Geometry: final body of the model. Coordinates: model frame, mm. Give positions to 0.01 mm unless a question says otherwise; leave off trailing zeros. Loops run counter-clockwise (first coordinate to the right, second up) from the corner with the lowest first, then second, coordinate; pieces in that order, holes last.
from build123d import *

# Parameters (mm, degrees)
SKETCH1_W               = 544
SKETCH1_H               = 376
BOSS_EXTRUDE1_DEPTH     = 5
SKETCH2_R               = 6.5
SKETCH2_R_2             = 3
F_1_JOYYSTICK_DEPTH     = 6
SKETCH3_R               = 12.5
F_1_BUTTONS_DEPTH       = 6
SKETCH4_R               = 6.75
F_1_ROCKET_SWITCH_DEPTH = 6
SKETCH5_R               = 2.4
SKETCH5_W               = 2
SKETCH5_H               = 74
F_1_POTENTIOMETER_DEPTH = 6
FILLET1_R               = 35
SKETCH6_R               = 12.5
F_2_BUTTONS_DEPTH       = 6
SKETCH9_R               = 25
F_2_SPEAKER_DEPTH       = 6
SKETCH8_R               = 2.4
SKETCH8_W               = 2
SKETCH8_H               = 75
F_2_POTENTIOMETER_DEPTH = 6
SKETCH11_R              = 1.8
F_2_PCB1_DEPTH          = 6
SKETCH12_R              = 1.8
F_1_PCB2_DEPTH          = 6
SKETCH13_R              = 1.8
F_2_USB_CONNECTOR_DEPTH = 6
SKETCH14_R              = 1.8
F_1_USB_CONNECTOR_DEPTH = 6
SKETCH15_R              = 3
POWER_DEPTH             = 6
SKETCH16_R              = 1.8
LED_FIXINGS_DEPTH       = 6
SKETCH10_R              = 6.75
CUT_EXTRUDE1_DEPTH      = 6


with BuildPart() as part:
    # Sketch1 → Boss-Extrude1 (new body)
    with BuildSketch(Plane(origin=(0, 0, 0), x_dir=(1, 0, 0), z_dir=(0, 1, 0))):
        with Locations((272, 188)):
            Rectangle(SKETCH1_W, SKETCH1_H)
    extrude(amount=BOSS_EXTRUDE1_DEPTH)

    # Sketch2 → 1 Joyystick (cut, through all)
    with BuildSketch(Plane(origin=(0, 5, 0), x_dir=(1, 0, 0), z_dir=(0, 1, 0))):
        with Locations((100, 276)):
            Circle(SKETCH2_R)
        with Locations((140.91, 297.59)):
            Circle(SKETCH2_R_2)
        with Locations((140.91, 254.41)):
            Circle(SKETCH2_R_2)
        with Locations((59.09, 254.41)):
            Circle(SKETCH2_R_2)
        with Locations((59.09, 297.59)):
            Circle(SKETCH2_R_2)
    extrude(amount=-F_1_JOYYSTICK_DEPTH, mode=Mode.SUBTRACT)

    # Sketch3 → 1 Buttons (cut, through all)
    with BuildSketch(Plane(origin=(0, 5, 0), x_dir=(1, 0, 0), z_dir=(0, 1, 0))):
        with Locations((60, 198)):
            Circle(SKETCH3_R)
        with Locations((110, 198)):
            Circle(SKETCH3_R)
        with Locations((80, 148)):
            Circle(SKETCH3_R)
        with Locations((130, 148)):
            Circle(SKETCH3_R)
        with Locations((130, 96)):
            Circle(SKETCH3_R)
    extrude(amount=-F_1_BUTTONS_DEPTH, mode=Mode.SUBTRACT)

    # Sketch4 → 1 Rocket Switch (cut, through all)
    with BuildSketch(Plane(origin=(0, 5, 0), x_dir=(1, 0, 0), z_dir=(0, 1, 0))):
        with Locations((180, 316)):
            Circle(SKETCH4_R)
    extrude(amount=-F_1_ROCKET_SWITCH_DEPTH, mode=Mode.SUBTRACT)

    # Sketch5 → 1 Potentiometer (cut, through all)
    with BuildSketch(Plane(origin=(0, 5, 0), x_dir=(1, 0, 0), z_dir=(0, 1, 0))):
        with Locations((178.719749064, 218)):
            Circle(SKETCH5_R)
        with Locations((192.718338039, 217.801237073)):
            Circle(SKETCH5_R)
        with Locations((192.718338039, 134.198762927)):
            Circle(SKETCH5_R)
        with Locations((178.719749064, 134)):
            Circle(SKETCH5_R)
        with Locations((191, 176)):
            Rectangle(SKETCH5_W, SKETCH5_H)
    extrude(amount=-F_1_POTENTIOMETER_DEPTH, mode=Mode.SUBTRACT)

    # Fillet1
    fillet1_edges = [part.edges().sort_by_distance(p)[0] for p in [
        (0, 2.5, -376),
        (544, 2.5, -376),
        (544, 2.5, 0),
        (0, 2.5, 0),
    ]]
    fillet(fillet1_edges, radius=FILLET1_R)

    # Sketch6 → 2 Buttons (cut, through all)
    with BuildSketch(Plane(origin=(0, 5, 0), x_dir=(1, 0, 0), z_dir=(0, 1, 0))):
        with Locations((484, 248)):
            Circle(SKETCH6_R)
        with Locations((404, 248)):
            Circle(SKETCH6_R)
        with Locations((484, 128)):
            Circle(SKETCH6_R)
        with Locations((404, 128)):
            Circle(SKETCH6_R)
        with Locations((444, 188)):
            Circle(SKETCH6_R)
    extrude(amount=-F_2_BUTTONS_DEPTH, mode=Mode.SUBTRACT)

    # Sketch9 → 2 speaker (cut, through all)
    with BuildSketch(Plane(origin=(0, 5, 0), x_dir=(1, 0, 0), z_dir=(0, 1, 0))):
        with Locations((444, 296)):
            Circle(SKETCH9_R)
    extrude(amount=-F_2_SPEAKER_DEPTH, mode=Mode.SUBTRACT)

    # Sketch8 → 2 Potentiometer (cut, through all)
    with BuildSketch(Plane(origin=(0, 5, 0), x_dir=(1, 0, 0), z_dir=(0, 1, 0))):
        with Locations((365, 218.5)):
            Circle(SKETCH8_R)
        with Locations((365, 133.5)):
            Circle(SKETCH8_R)
        with Locations((351, 133.5)):
            Circle(SKETCH8_R)
        with Locations((351, 218.5)):
            Circle(SKETCH8_R)
        with Locations((353, 176)):
            Rectangle(SKETCH8_W, SKETCH8_H)
    extrude(amount=-F_2_POTENTIOMETER_DEPTH, mode=Mode.SUBTRACT)

    # Sketch11 → 2 PCB1 (cut, through all)
    with BuildSketch(Plane(origin=(0, 5, 0), x_dir=(1, 0, 0), z_dir=(0, 1, 0))):
        with Locations((374, 96)):
            Circle(SKETCH11_R)
        with Locations((314, 96)):
            Circle(SKETCH11_R)
        with Locations((314, 296)):
            Circle(SKETCH11_R)
        with Locations((374, 296)):
            Circle(SKETCH11_R)
    extrude(amount=-F_2_PCB1_DEPTH, mode=Mode.SUBTRACT)

    # Sketch12 → 1 PCB2 (cut, through all)
    with BuildSketch(Plane(origin=(0, 5, 0), x_dir=(1, 0, 0), z_dir=(0, 1, 0))):
        with Locations((230, 96)):
            Circle(SKETCH12_R)
        with Locations((170, 96)):
            Circle(SKETCH12_R)
        with Locations((230, 296)):
            Circle(SKETCH12_R)
        with Locations((170, 296)):
            Circle(SKETCH12_R)
    extrude(amount=-F_1_PCB2_DEPTH, mode=Mode.SUBTRACT)

    # Sketch13 → 2 USB Connector (cut, through all)
    with BuildSketch(Plane(origin=(0, 5, 0), x_dir=(1, 0, 0), z_dir=(0, 1, 0))):
        with Locations((384, 50)):
            Circle(SKETCH13_R)
        with Locations((357, 50)):
            Circle(SKETCH13_R)
    extrude(amount=-F_2_USB_CONNECTOR_DEPTH, mode=Mode.SUBTRACT)

    # Sketch14 → 1 USB Connector (cut, through all)
    with BuildSketch(Plane(origin=(0, 5, 0), x_dir=(1, 0, 0), z_dir=(0, 1, 0))):
        with Locations((187, 50)):
            Circle(SKETCH14_R)
        with Locations((160, 50)):
            Circle(SKETCH14_R)
    extrude(amount=-F_1_USB_CONNECTOR_DEPTH, mode=Mode.SUBTRACT)

    # Sketch15 → Power (cut, through all)
    with BuildSketch(Plane(origin=(0, 5, 0), x_dir=(1, 0, 0), z_dir=(0, 1, 0))):
        with Locations((230, 326)):
            Circle(SKETCH15_R)
    extrude(amount=-POWER_DEPTH, mode=Mode.SUBTRACT)

    # Sketch16 → LED fixings (cut, through all)
    with BuildSketch(Plane(origin=(0, 5, 0), x_dir=(1, 0, 0), z_dir=(0, 1, 0))):
        with Locations((517, 30)):
            Circle(SKETCH16_R)
        with Locations((327, 30)):
            Circle(SKETCH16_R)
        with Locations((517, 346)):
            Circle(SKETCH16_R)
        with Locations((327, 346)):
            Circle(SKETCH16_R)
        with Locations((217, 346)):
            Circle(SKETCH16_R)
        with Locations((27, 346)):
            Circle(SKETCH16_R)
        with Locations((217, 30)):
            Circle(SKETCH16_R)
        with Locations((27, 30)):
            Circle(SKETCH16_R)
    extrude(amount=-LED_FIXINGS_DEPTH, mode=Mode.SUBTRACT)

    # Sketch10 → Cut-Extrude1 (cut, through all)
    with BuildSketch(Plane(origin=(0, 5, 0), x_dir=(1, 0, 0), z_dir=(0, 1, 0))):
        with Locations((364, 316)):
            Circle(SKETCH10_R)
    extrude(amount=-CUT_EXTRUDE1_DEPTH, mode=Mode.SUBTRACT)


solid = part.part
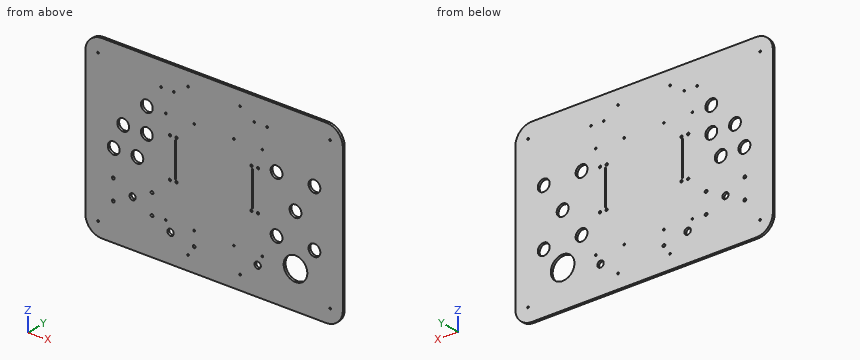
Item 1: Section query C-C on y = 4.05. Give the number of separate pieces and of enclosed holes in the cut face, plus the area to 3 significant figures.
Values follow:
separate pieces: 1
enclosed holes: 49
area: 195,000 mm2
Item 2: Ray query, probe 1 along Z at (x, y) = (365, 1.75); probe 2 along X at (y, z) = (2.35, -149.5); probe 3 along Z at (x, y) = (229.5, 1.15). Return the intervals inside material, ascending.
Values follow:
probe 1: z = -376 to -322.68, -309.32 to -220.9, -216.1 to -135.9, -131.1 to 0
probe 2: x = 0 to 67.59, 92.41 to 117.59, 142.41 to 190, 192 to 352, 354 to 544
probe 3: z = -376 to -328.96, -323.04 to -297.73, -294.27 to -97.73, -94.27 to 0
Item 3: Section query A-A on x = 130. Return loops of the section in (y, z).
Values follow:
outline: (0, -376) - (5, -376) - (5, -160.5) - (0, -160.5) - close; (0, -135.5) - (5, -135.5) - (5, -108.5) - (0, -108.5) - close; (0, -83.5) - (5, -83.5) - (5, 0) - (0, 0) - close
Item 4: Section query B-B on x = 425.5. Return loops of the section in (y, z), plus the area to 3 significant figures.
Values follow:
outline: (0, -376) - (5, -376) - (5, -312.82) - (0, -312.82) - close; (0, -279.18) - (5, -279.18) - (5, 0) - (0, 0) - close
area: 1,710 mm2
